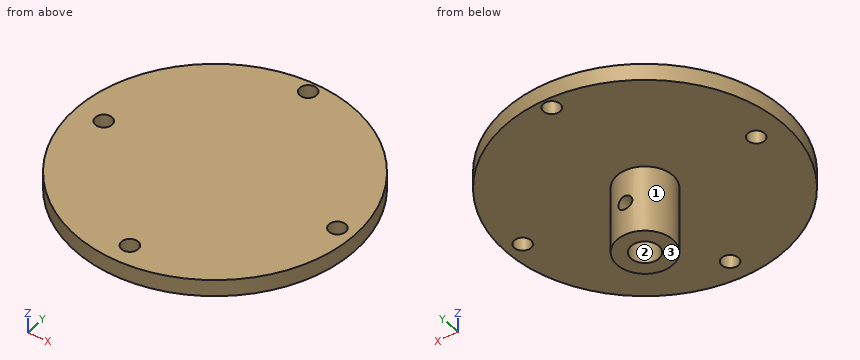
```python
from build123d import *

# Parameters (mm, degrees)
SZKIC1_R                        = 25
DODANIE_WYCI_GNI_CIE1_DEPTH     = 3
SZKIC2_R                        = 5
SZKIC2_R_2                      = 2.5
DODANIE_WYCI_GNI_CIE2_DEPTH     = 12
WYTNIJ_WYCI_GNI_CIE1_REACH      = 39.336
WYTNIJ_WYCI_GNI_CIE1_END_RADIUS = 5
SZKIC3_R                        = 1.25
WYTNIJ_WYCI_GNI_CIE2_REACH      = 40.406
SZKIC4_R                        = 1.5


with BuildPart() as part:
    # Szkic1 → Dodanie-wyciągnięcie1 (new body)
    with BuildSketch(Plane.XY):
        Circle(SZKIC1_R)
    extrude(amount=DODANIE_WYCI_GNI_CIE1_DEPTH)

    # Szkic2 → Dodanie-wyciągnięcie2 (add)
    with BuildSketch(Plane(origin=(0, 0, 0), x_dir=(-1, 0, 0), z_dir=(0, 0, -1))):
        Circle(SZKIC2_R)
        Circle(SZKIC2_R_2, mode=Mode.SUBTRACT)
    extrude(amount=DODANIE_WYCI_GNI_CIE2_DEPTH)

    # Wytnij-wyciągnięcie1: up to this cylinder (the profile starts inside it)
    wytnij_wyci_gni_cie1_end = Plane(origin=(0, 0, -6), z_dir=(0, 0, 1)) * Cylinder(WYTNIJ_WYCI_GNI_CIE1_END_RADIUS, 89.672, mode=Mode.PRIVATE)
    # Szkic3 → Wytnij-wyciągnięcie1 (cut, up to the surface)
    with BuildSketch(Plane(origin=(0, 0, 0), x_dir=(1, 0, 0), z_dir=(0, 1, 0)), mode=Mode.PRIVATE) as wytnij_wyci_gni_cie1_sk1:
        with Locations(Location((0, 6, 0), (0, 0, 90))):
            Circle(SZKIC3_R)
    wytnij_wyci_gni_cie1_tool1 = extrude(wytnij_wyci_gni_cie1_sk1.sketch, amount=WYTNIJ_WYCI_GNI_CIE1_REACH, mode=Mode.PRIVATE) & wytnij_wyci_gni_cie1_end
    add(wytnij_wyci_gni_cie1_tool1.solids().sort_by_distance((0, 0, -6))[0], mode=Mode.SUBTRACT)

    # Szkic4 → Wytnij-wyciągnięcie2 (cut, up to next)
    with BuildSketch(Plane.XY.offset(3), mode=Mode.PRIVATE) as wytnij_wyci_gni_cie2_sk1:
        with Locations((22, 0)):
            Circle(SZKIC4_R)
    wytnij_wyci_gni_cie2_tool1 = extrude(wytnij_wyci_gni_cie2_sk1.sketch, amount=-WYTNIJ_WYCI_GNI_CIE2_REACH, mode=Mode.PRIVATE) & part.part
    # Szkic4 → Wytnij-wyciągnięcie2 (cut, up to next)
    with BuildSketch(Plane.XY.offset(3), mode=Mode.PRIVATE) as wytnij_wyci_gni_cie2_sk2:
        with Locations((-20, 0)):
            Circle(SZKIC4_R)
    wytnij_wyci_gni_cie2_tool2 = extrude(wytnij_wyci_gni_cie2_sk2.sketch, amount=-WYTNIJ_WYCI_GNI_CIE2_REACH, mode=Mode.PRIVATE) & part.part
    # Szkic4 → Wytnij-wyciągnięcie2 (cut, up to next)
    with BuildSketch(Plane.XY.offset(3), mode=Mode.PRIVATE) as wytnij_wyci_gni_cie2_sk3:
        with Locations((0, -21)):
            Circle(SZKIC4_R)
    wytnij_wyci_gni_cie2_tool3 = extrude(wytnij_wyci_gni_cie2_sk3.sketch, amount=-WYTNIJ_WYCI_GNI_CIE2_REACH, mode=Mode.PRIVATE) & part.part
    # Szkic4 → Wytnij-wyciągnięcie2 (cut, up to next)
    with BuildSketch(Plane.XY.offset(3), mode=Mode.PRIVATE) as wytnij_wyci_gni_cie2_sk4:
        with Locations((0, 23)):
            Circle(SZKIC4_R)
    wytnij_wyci_gni_cie2_tool4 = extrude(wytnij_wyci_gni_cie2_sk4.sketch, amount=-WYTNIJ_WYCI_GNI_CIE2_REACH, mode=Mode.PRIVATE) & part.part
    add(wytnij_wyci_gni_cie2_tool1.solids().sort_by_distance((22, 0, 3))[0], mode=Mode.SUBTRACT)
    add(wytnij_wyci_gni_cie2_tool2.solids().sort_by_distance((-20, 0, 3))[0], mode=Mode.SUBTRACT)
    add(wytnij_wyci_gni_cie2_tool3.solids().sort_by_distance((0, -21, 3))[0], mode=Mode.SUBTRACT)
    add(wytnij_wyci_gni_cie2_tool4.solids().sort_by_distance((0, 23, 3))[0], mode=Mode.SUBTRACT)


solid = part.part
```
Check sheet for the modelled part. Datum: model origin and axes. Units: mm. Face numbers are marked on the shaded views. Round coordinates to 2 decimals unless told otherwise and drop trailing zeros. Order: outer loops, then holes, each group sorted by start corner. A loop starts at its lowest first (then second) coordinate and runs counter-clockwise, first axis right, second up. Notation, with made-up numbers: (-8, -36) -> (10, -36) arc R14 cw to (10, -10) -> close; hole circle Ø2 at (80.25, 42). An arc over 180 degrees is marked (long way). One line per item, written item: value. Start each with the question number.
Q1. Cross-section at C-C (x = 0). Record the boundary of the cut face in (y, z).
Q2. Cross-section at D-D (z = -1.5). Record the boundary of the cut face in (x, y), and give its area (3 significant figures).
Q3. Gauge pin test, flat ends, axial feed: pin 1 Ø3 at (x, z) = (0, -6) entering from +Y; pin 2 Ø1.5 at (x, z) = (0.5, 0) entering from -Y; pin 3 Ø1.5 at (x, y) = (0, -0.5) entering from -Z. Record the tip position at first contact, or that the pin passes through.
Q4. Cross-section at A-A (x = -20). Record the boundary of the cut face in (y, z), and give its area (3 significant figures).
Q5. Mould release check, pull along Y, two halves, no side actions. Record for the marked faces 1, 2 and 3: pulls with the +Y half, pulls with the -Y half, needs draft (parallel to the pull), parting line crosses it, or undercut.
Q6. Thickness scan on line 1 (Y direction, x = 0, z = 1.7); line 2 (Z direction, x = 9.5, y = 5); line 3 (Y direction, x = -20, z = 0.9). Record the ranges inside material, lowest first.
Q7. Cross-section at B-B (y = 0). Record the boundary of the cut face in (x, z), and give its area (3 significant figures).
Completed:
1. outline: (-25, 0) -> (-22.5, 0) -> (-22.5, 3) -> (-25, 3) -> close; (-19.5, 0) -> (-5, 0) -> (-5, -12) -> (-2.5, -12) -> (-2.5, 0) -> (2.5, 0) -> (2.5, -4.75) -> (5, -4.75) -> (5, 0) -> (21.5, 0) -> (21.5, 3) -> (-19.5, 3) -> close; (2.5, -12) -> (5, -12) -> (5, -7.25) -> (2.5, -7.25) -> close; (24.5, 0) -> (25, 0) -> (25, 3) -> (24.5, 3) -> close
2. outline: circle Ø10 at (0, 0); hole circle Ø5 at (0, 0)
2. area: 58.9 mm²
3. pin 1: stops at y = 5
3. pin 2: stops at y = -25
3. pin 3: stops at z = 0
4. outline: (-15, 0) -> (-1.5, 0) -> (-1.5, 3) -> (-15, 3) -> close; (1.5, 0) -> (15, 0) -> (15, 3) -> (1.5, 3) -> close
4. area: 81.0 mm²
5. face 1: parting line crosses it
5. face 2: undercut
5. face 3: needs draft
6. line 1: y = -25 to -22.5, -19.5 to 21.5, 24.5 to 25
6. line 2: z = 0 to 3
6. line 3: y = -15 to -1.5, 1.5 to 15
7. outline: (-25, 0) -> (-21.5, 0) -> (-21.5, 3) -> (-25, 3) -> close; (-18.5, 0) -> (-5, 0) -> (-5, -12) -> (-2.5, -12) -> (-2.5, 0) -> (2.5, 0) -> (2.5, -12) -> (5, -12) -> (5, 0) -> (20.5, 0) -> (20.5, 3) -> (-18.5, 3) -> close; (23.5, 0) -> (25, 0) -> (25, 3) -> (23.5, 3) -> close
7. area: 192 mm²
